For this review, take the finished solid that the model builds, in its own axes (mm). A direction names the side the tool comes from. Give positions to 0.01 mm unless a question says otherwise; leave off trailing zeros. Loops run counter-clockwise (first coordinate to the right, second up) from the corner with the lowest first, then second, coordinate; pieces in that order, holes last. Notation, with made-up numbers: (-25.75, -16.5) - (-8.75, -16.5) arc R16 cw to (-8.75, -1.5) - close; hole circle Ø7 at (37, 24.25). An arc over 180 degrees is marked (long way). Put each result on its own line as item: value.
from build123d import *

# Parameters (mm, degrees)
F0_W     = 156.9848433137
F0_H     = 92.025604099
F1_DEPTH = 25.4
F2_W     = 135.7623711228
F2_H     = 72.5497286767
F4_DEPTH = 127
F6_D     = 25.4
F8_R     = 16.8146432666
F9_DEPTH = 72.5497286767


# Not quite as in the source:
# - a feature of the source that left no trace in its solid (it failed there, or was rolled back) is left out


with BuildPart() as f1:
    # F0 (on Right) → F1 (new body)
    with BuildSketch(Plane.YZ):
        with Locations((14.6216116846, 4.5173931867)):
            Rectangle(F0_W, F0_H)
    extrude(amount=F1_DEPTH)

    # F2 (on Front) → F4 (join)
    with BuildSketch(Plane.XZ):
        with Locations((-2.4367310107, -7.2724418715)):
            Rectangle(F2_W, F2_H)
    extrude(amount=F4_DEPTH)

    # F6 (through all)
    with Locations(Plane(origin=(0, 0, -43.5473062098), x_dir=(1, 0, 0), z_dir=(0, 0, -1))):
        with Locations((38.019452244, 112.0775043964), (38.019452244, 35.0753962994), (-26.6502853483, 35.0753962994), (-26.6502853483, 112.0775043964)):
            Hole(F6_D / 2)

    # F8 (on face) → F9 (cut, through all)
    with BuildSketch(Plane(origin=(0, 0, -43.5473062098), x_dir=(1, 0, 0), z_dir=(0, 0, -1))):
        with Locations((6.7373481579, 78.689865768)):
            Circle(F8_R)
    extrude(amount=-F9_DEPTH, mode=Mode.SUBTRACT)


solid = f1.part
1) Take a section at B-B on x = 48.5. State the section outline as (y, z) points, and give its area (3 significant figures).
Geometry check:
outline: (-127, -43.55) - (-119.25, -43.55) - (-119.25, 29) - (-127, 29) - close; (-104.9, -43.55) - (-42.25, -43.55) - (-42.25, 29) - (-104.9, 29) - close; (-27.9, -43.55) - (0, -43.55) - (0, 29) - (-27.9, 29) - close
area: 7,130 mm²
2) Take a section at A-A on y = -105. State the section outline as (x, z) points, and give its area (3 significant figures).
Geometry check:
outline: (-70.32, -43.55) - (-37.2, -43.55) - (-37.2, 29) - (-70.32, 29) - close; (-16.11, -43.55) - (27.47, -43.55) - (27.47, 29) - (-16.11, 29) - close; (48.56, -43.55) - (65.44, -43.55) - (65.44, 29) - (48.56, 29) - close
area: 6,790 mm²
3) Draft analysis for pull direction Y (two halves, no side actions). For faces 1 (the face through (13, 46, -41.495)), 2 (the face through (13, -63.871, 40)), 3 (the face through (22.776, -83.741, -7.78)), state which applies: pulls with the +Y half, pulls with the -Y half, needs draft (parallel to the pull), parting line crosses it, or undercut.
Geometry check:
face 1: needs draft
face 2: pulls with the -Y half
face 3: undercut
4) Wall thickness on line 1 (X direction, y = -112.5, z = -37.5); line 2 (Y direction, x = -16, z = 1); line 3 (Y direction, x = -25.5, z = 19.5): over which ranges is each line inside the solid? List them lowest first.
Geometry check:
line 1: x = -70.32 to -39.34, -13.96 to 25.33, 50.71 to 65.44
line 2: y = -127 to -119, -105.16 to -41.99, -28.16 to 0
line 3: y = -127 to -124.73, -99.43 to -47.72, -22.43 to 0
5) Insertion check: pin 1 Ø7.5 at (x, y) = (18, 65) entering from -Z; pin 2 Ø6.5 at (y, z) = (-47.5, 37) entering from +X; pin 3 Ø4 at (x, z) = (3.5, 32.5) entering from -Y; pin 4 Ø23 at (x, y) = (38.02, -112.08) entering from +Z. Each pin has a flat end and moves straight along its axis. Give the tip position at first contact, or say it passes through.
Geometry check:
pin 1: stops at z = -41.5
pin 2: stops at x = 25.4
pin 3: stops at y = -63.87
pin 4: passes through
6) Take a section at D-D on x = 19. State the section outline as (y, z) points.
Geometry check:
outline: (-127, -43.55) - (-90.19, -43.55) - (-90.19, 29) - (-127, 29) - close; (-67.19, -43.55) - (0, -43.55) - (0, -41.5) - (93.11, -41.5) - (93.11, 50.53) - (-63.87, 50.53) - (-63.87, 29) - (-67.19, 29) - close
7) Take a section at C-C on z = -4.5. State the section outline as (x, y) points.
Geometry check:
outline: (-70.32, -127) - (65.44, -127) - (65.44, 0) - (25.4, 0) - (25.4, 93.11) - (0, 93.11) - (0, 0) - (-70.32, 0) - close; hole circle Ø25.4 at (-26.65, -112.08); hole circle Ø25.4 at (-26.65, -35.08); hole circle Ø33.63 at (6.74, -78.69); hole circle Ø25.4 at (38.02, -112.08); hole circle Ø25.4 at (38.02, -35.08)
8) For faces 4 (the face through (-38.764, -38.89, -6.765)), 5 (the face through (25.4, -50, 40)), list the 3-axis set-ups (+Z, -Z, +X, -X, +Y, -Y) from which the entire face can be reached by the end or side of a thin tool; tool diameter is ignored.
Geometry check:
face 4: +Z, -Z
face 5: +Z, +X, +Y, -Y
